Part model, mm, in its own coordinate system. Face numbers are marked on the shaded views. A direction names the side the tool comes from. Coordinates: 2 decimals unless noted, no trailing zeros. Order: outer loops, then holes, each group sorted by start corner. A loop starts at its lowest first (then second) coordinate and runs counter-clockwise, first axis right, second up.
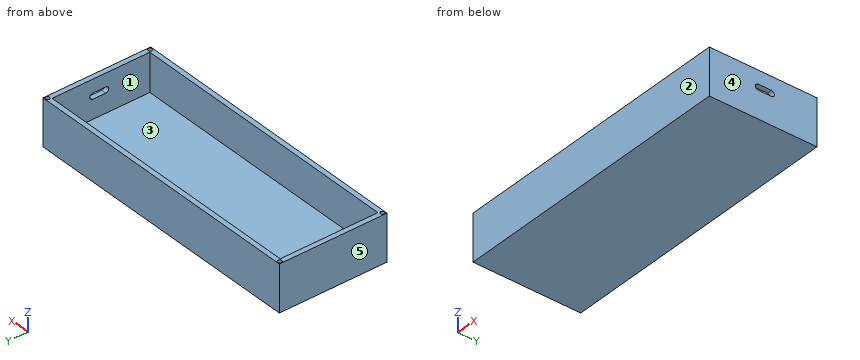
from build123d import *

# Parameters (mm, degrees)
SKETCH1_W           = 174
SKETCH1_H           = 65
BOSS_EXTRUDE1_DEPTH = 5
SKETCH3_W           = 174
SKETCH3_H           = 65
SKETCH3_W_2         = 168
SKETCH3_H_2         = 59
BOSS_EXTRUDE3_DEPTH = 23
CUT_EXTRUDE1_DEPTH  = 23
SKETCH17_R          = 1.25
CUT_EXTRUDE5_DEPTH  = 4
SKETCH15_R          = 1.25
CUT_EXTRUDE4_DEPTH  = 4
SKETCH11_R          = 1.25
SKETCH11_R_2        = 0.084381571
CUT_EXTRUDE2_DEPTH  = 4
SKETCH13_R          = 0.084381571
CUT_EXTRUDE3_DEPTH  = 4


with BuildPart() as part:
    # Sketch1 → Boss-Extrude1 (new body)
    with BuildSketch(Plane.XY):
        Rectangle(SKETCH1_W, SKETCH1_H)
    extrude(amount=BOSS_EXTRUDE1_DEPTH)

    # Sketch3 → Boss-Extrude3 (add)
    with BuildSketch(Plane.XY.offset(5)):
        Rectangle(SKETCH3_W, SKETCH3_H)
        Rectangle(SKETCH3_W_2, SKETCH3_H_2, mode=Mode.SUBTRACT)
    extrude(amount=BOSS_EXTRUDE3_DEPTH)

    # Sketch9 → Cut-Extrude1 (cut)
    with BuildSketch(Plane(origin=(87, 0, 0), x_dir=(0, 0, -1), z_dir=(1, 0, 0))):
        with BuildLine():
            Line((-20, -3), (-20, 5))
            ThreePointArc((-20, 5), (-18.25, 6.75), (-16.5, 5))
            Line((-16.5, 5), (-16.5, -3))
            ThreePointArc((-16.5, -3), (-18.25, -4.75), (-20, -3))
        make_face()
    extrude(amount=-CUT_EXTRUDE1_DEPTH, mode=Mode.SUBTRACT)

    # Sketch17 → Cut-Extrude5 (cut)
    with BuildSketch(Plane.XY.offset(28)):
        with Locations((-85.5, -31)):
            Circle(SKETCH17_R)
        with Locations((-85.5, 31)):
            Circle(SKETCH17_R)
        with Locations((85.5, 31)):
            Circle(SKETCH17_R)
        with Locations((85.5, -31)):
            Circle(SKETCH17_R)
    extrude(amount=-CUT_EXTRUDE5_DEPTH, mode=Mode.SUBTRACT)

    # Sketch15 → Cut-Extrude4 (cut)
    with BuildSketch(Plane.XY.offset(28)):
        with Locations((-85.5, 31)):
            Circle(SKETCH15_R)
    extrude(amount=-CUT_EXTRUDE4_DEPTH, mode=Mode.SUBTRACT)

    # Sketch11 → Cut-Extrude2 (cut)
    with BuildSketch(Plane.XY.offset(28)):
        with Locations((-85.5, 31)):
            Circle(SKETCH11_R)
        with Locations((-85.5, 31)):
            Circle(SKETCH11_R_2, mode=Mode.SUBTRACT)
    extrude(amount=-CUT_EXTRUDE2_DEPTH, mode=Mode.SUBTRACT)

    # Sketch13 → Cut-Extrude3 (cut)
    with BuildSketch(Plane.XY.offset(28)):
        with Locations((-85.5, 31)):
            Circle(SKETCH13_R)
    extrude(amount=-CUT_EXTRUDE3_DEPTH, mode=Mode.SUBTRACT)


solid = part.part
Q1. Which spindle directions (+Z, -Z, +X, -X, +Y, -Y) get a long thin tool onto all of the face, cutting with end or side? Do the marked faces 1 and 2. Say none if no direction does.
Results list:
face 1: +Z
face 2: +Z, -Z, +X, -X, -Y
Q2. Cut at B-B on z = 12.25. Write the cut outline in (x, y), and give its area (3 significant figures).
Results list:
outline: (-87, -32.5) - (87, -32.5) - (87, 32.5) - (-87, 32.5) - close; hole (-84, -29.5) - (84, -29.5) - (84, 29.5) - (-84, 29.5) - close
area: 1,400 mm2
Q3. Cut at A-A on x = -29. Write the cut outline in (y, z), and give its area (3 significant figures).
Results list:
outline: (-32.5, 0) - (32.5, 0) - (32.5, 28) - (29.5, 28) - (29.5, 5) - (-29.5, 5) - (-29.5, 28) - (-32.5, 28) - close
area: 463 mm2
Q4. Mould opens along X. For the marked faces 3, 4 and 5 say: pulls with the +X half, pulls with the -X half, needs draft (parallel to the pull), parting line crosses it, or undercut.
Results list:
face 3: undercut
face 4: pulls with the +X half
face 5: pulls with the -X half
Q5. Pin check, flat tip, straight feed: pin 1 Ø2 at (x, y) = (-85.5, 31) entering from +Z. Stop position of the tip, or through.
Results list:
pin 1: stops at z = 24
Q6. Wall check: line 1 along Y through (x, z) = (85.5, 25.1); line 2 along Y through (x, z) = (-37, 21.75); line 3 along X through (y, z) = (10, 13.75). Give the ranges that are in metal, low to high.
Results list:
line 1: y = -32.5 to -32.25, -29.75 to 29.75, 32.25 to 32.5
line 2: y = -32.5 to -29.5, 29.5 to 32.5
line 3: x = -87 to -84, 84 to 87
Q7. Cut at C-C on y = 21. Write the cut outline in (x, z), and give its area (3 significant figures).
Results list:
outline: (-87, 0) - (87, 0) - (87, 28) - (84, 28) - (84, 5) - (-84, 5) - (-84, 28) - (-87, 28) - close
area: 1,010 mm2
